Could you check a few things on this model? Use its own coordinates, in mm. Face numbers are marked on the shaded views. A direction names the side the tool comes from. Coordinates: 2 decimals unless noted, no trailing zeros. Write each loop counter-clockwise with the first axis right and the second up, starting at its lowest first coordinate (ties: lowest second). Pieces come first, ordered by that corner, then holes. Notation, with made-up numbers: M 70.25,-26.5 L 110.25,-26.5 A22 cw 110.25,-18.5 Z; hole C 49,72.25 d3. An arc over 180 degrees is marked long. Answer as CSV lines item,"result". Start each with the question number.
Item 1: If I drill on line 1 along Z through (x, y) = (0, 3.5); line 2 along X through (y, z) = (5.25, -5) (3 decimals); line 3 along X through (y, z) = (6.5, -11), over which ranges is the centre line in solid material (lowest first)? Write a range as [from, to].
Item 2: We'd pull the mould along Z, two halves only. Please class the marked faces 1, 2, 3 and 4: +Z half, -Z half, draft (parallel to the pull), parting line (faces both ways), or undercut.
Item 3: Suppose I cut it at D-D, the plane x = -3. Write out the boundary of the cut face in (y, z).
Item 4: On a 3-axis mill with a long thin cutter (end or side, diameter ignored), from which of +Z, -Z, +X, -X, +Y, -Y can I reach the whole of each face in a straight line? I mean the marked faces 5 and 6. Say none if no direction works.
Item 5: I'm going to push flat-ended pins straight in: P1, Ø2, axis at x = 4.5, y = 6, coming from the +Z side; P2, Ø3, axis at x = 7.5, z = 19.5, coming from the -Y side. Where does each tip first touch, or does it pass through?
Item 6: Suppose I cut it at C-C, the plane x = 0.5. Write out the boundary of the cut face in (y, z).
Item 7: Suppose I cut it at B-B, the plane z = -10.5. Write out the boundary of the cut face in (x, y), and give its area (3 significant figures).
Item 8: Suppose I cut it at A-A, the plane y = 1.75. Write out the boundary of the cut face in (x, z), and give its area (3 significant figures).
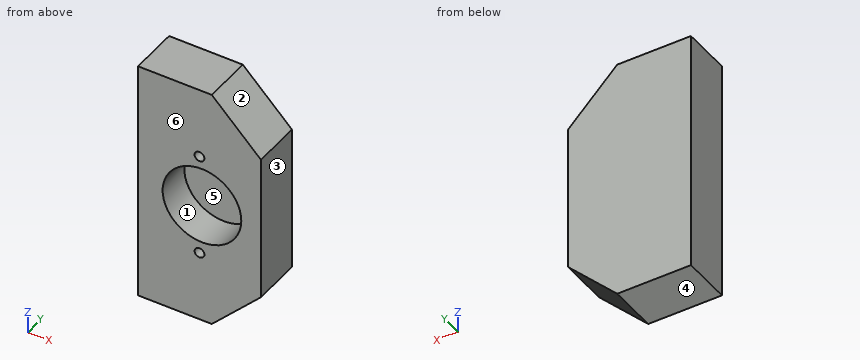
Autodesk Inventor part; units mm, degrees
ref_plane "YZ Plane" through (0, 0, 0) normal (1, 0, 0) x (0, 1, 0)
ref_plane "XZ Plane" through (0, 0, 0) normal (0, 1, 0) x (-1, 0, 0)
ref_plane "XY Plane" through (0, 0, 0) normal (0, 0, 1) x (1, 0, 0)
sketch "스케치1" plane through (0, 0, 0) normal (0, 1, 0) x (-1, 0, 0)
  line L0 (12.5, 25) -> (-12.5, 25)
  line L1 (-12.5, 25) -> (-12.5, -25)
  line L2 (-12.5, -25) -> (12.5, -25)
  line L3 (12.5, -25) -> (12.5, 25)
  line L4 (12.5, 25) -> (-12.5, -25) construction
  line L5 (-12.5, 25) -> (12.5, -25) construction
  point P0 (0, 0)
  dimension "d0" = 50
  dimension "d1" = 25
extrude "돌출1" add sketch "스케치1" along normal blind 10
chamfer "모따기1" distance 10 angle 45 2 edges at (12.5, 5, -25) (12.5, 5, 25)
sketch "스케치2" plane through (0, 0, 0) normal (0, -1, 0) x (1, 0, 0)
  circle A0 centre (0.5, 0) radius 8
  line L0 (12.5, 15) -> (12.5, -15)
  point P0 (0, 0)
  point P1 (12.5, 0)
  point P2 (12.5, 0)
  dimension "d7" = 16
  dimension "d8" = 12
extrude "돌출2" cut sketch "스케치2" against normal blind 7
sketch "스케치3" plane through (0, 0, 0) normal (0, -1, 0) x (1, 0, 0)
  circle A0 centre (0, 10.5) radius 1
  line L0 (0, 0) -> (5.1796, 0)
  circle A1 centre (-10.5, 0) radius 1
  circle A2 centre (0, -10.5) radius 1
  circle A3 centre (10.5, 0) radius 1
  dimension "d11" = 2
  dimension "d18" = 360
  dimension "d20" = 21
extrude "돌출3" cut sketch "스케치3" against normal blind 7 contours A0 | A2
properties part number "책상 고정 판"
Ans:
1,line 1,"z = [-25, -11.5], [-9.5, -7.98], [7.98, 9.5], [11.5, 25]"
1,line 2,"x = [-12.5, -5.745], [6.745, 12.5]"
1,line 3,"x = [-12.5, -0.87], [0.87, 12.5]"
2,face 1,"undercut"
2,face 2,"+Z half"
2,face 3,"draft"
2,face 4,"-Z half"
3,outline,"M 0,-25 L 10,-25 L 10,25 L 0,25 L 0,7.19 L 7,7.19 L 7,-7.19 L 0,-7.19 Z"
4,face 5,"-Y"
4,face 6,"+Z, -Z, +X, -X, -Y"
5,P1,"stops at z = 24"
5,P2,"stops at y = 0"
6,outline,"M 0,-25 L 10,-25 L 10,25 L 0,25 L 0,11.37 L 7,11.37 L 7,9.63 L 0,9.63 L 0,8 L 7,8 L 7,-8 L 0,-8 L 0,-9.63 L 7,-9.63 L 7,-11.37 L 0,-11.37 Z"
7,outline,"M -12.5,0 L -1,0 L -1,7 L 1,7 L 1,0 L 12.5,0 L 12.5,10 L -12.5,10 Z"
7,area,"236 mm^2"
8,outline,"M -12.5,-25 L 2.5,-25 L 12.5,-15 L 12.5,15 L 2.5,25 L -12.5,25 Z; hole C 0.5,0 d16; hole C 0,-10.5 d2; hole C 0,10.5 d2"
8,area,"943 mm^2"
